Check sheet for the modelled part. Datum: model origin and axes. Units: mm. Give positions to 0.01 mm unless a question says otherwise; leave off trailing zeros. Loops run counter-clockwise (first coordinate to the right, second up) from the corner with the lowest first, then second, coordinate; pieces in that order, holes last. Notation, with made-up numbers: (86, -38.75) - (103, -38.75) arc R20 ccw to (103, -20.75) - close; hole circle Ø8 at (48, 47). An arc over 180 degrees is marked (long way). Use one line per item in the form item = value.
from build123d import *

# Parameters (mm, degrees)
F0_R     = 5
F1_DEPTH = 10


with BuildPart() as f1:
    # F0 (on Top) → F1 (new body)
    with BuildSketch(Plane.XY):
        Polygon((-195, 30), (-240, 10), (-240, -10), (-200, -27.777778), (-200, -52), (-150, -52), (-150, -308), (0, -308), (150, -308), (150, -52), (200, -52), (200, -27.777778), (240, -10), (240, 10), (195, 30), (195, 192), (0, 192), (-195, 192), align=None)
        with Locations((-175, -27)):
            Circle(F0_R, mode=Mode.SUBTRACT)
        with Locations((175, -27)):
            Circle(F0_R, mode=Mode.SUBTRACT)
    extrude(amount=F1_DEPTH)


solid = f1.part
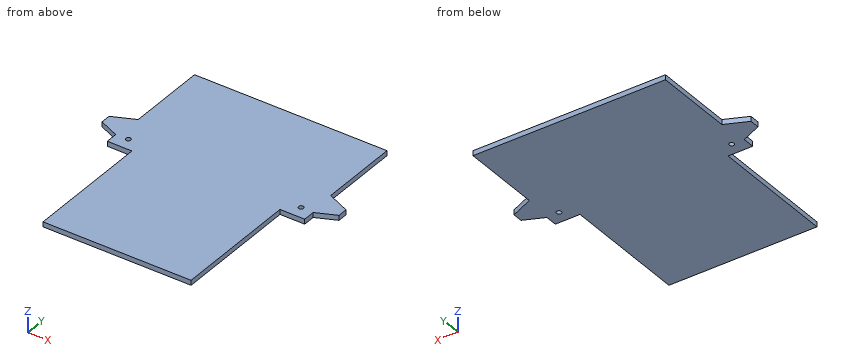
Item 1: Section check B-B on y = -110.5. Record the boundary of the cut face in (x, z), then the cut area to 3 significant figures.
Answer block:
outline = (-150, 0) - (150, 0) - (150, 10) - (-150, 10) - close
area = 3,000 mm2
Item 2: Section check A-A on z = 5.5. Record the boundary of the cut face in (x, y).
Answer block:
outline = (-240, -10) - (-200, -27.78) - (-200, -52) - (-150, -52) - (-150, -308) - (150, -308) - (150, -52) - (200, -52) - (200, -27.78) - (240, -10) - (240, 10) - (195, 30) - (195, 192) - (-195, 192) - (-195, 30) - (-240, 10) - close; hole circle Ø10 at (-175, -27); hole circle Ø10 at (175, -27)
Item 3: Thickness scan on L1, parallel to Y at x = 175, z = 3.75; L2, parallel to X at y = -25, z = 9.25; L3, parallel to Y at x = 188.5, z = 5. Record the ranges inside material, lowest first.
Answer block:
L1 = -52 to -32, -22 to 192
L2 = -206.25 to -179.58, -170.42 to 170.42, 179.58 to 206.25
L3 = -52 to 192
Item 4: Gauge pin test, flat ends, axial feed: P1, Ø3, axis at x = 172, z = 7, coming from the -Y side; P2, Ø9, axis at x = 175, y = -27, coming from the -Z side; P3, Ø5, axis at y = -181, z = 3.5, coming from the -X side; P4, Ø3, axis at y = -34.5, z = 5.5, coming from the +X side. Record the tip position at first contact, or that the pin passes through.
Answer block:
P1 = -52
P2 = through
P3 = -150
P4 = 200
